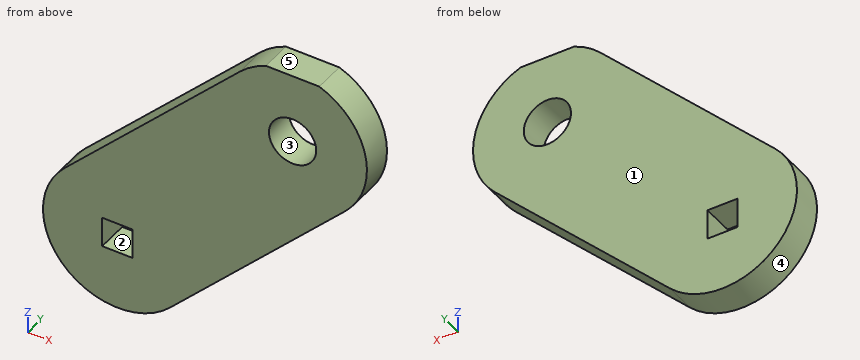
```python
from build123d import *

# Parameters (mm, degrees)
SKETCH2_R           = 4.7625
SKETCH2_W           = 6.1
SKETCH2_H           = 6.1
BOSS_EXTRUDE1_DEPTH = 6.35


with BuildPart() as part:
    # Sketch2 → Boss-Extrude1 (new body)
    with BuildSketch(Plane(origin=(0, 0, 0), x_dir=(1, 0, 0), z_dir=(0, 1, 0))):
        with BuildLine():
            Line((45.961940777, -24.748737342), (10.606601718, 10.606601718))
            ThreePointArc((10.606601718, 10.606601718), (-10.606601718, 10.606601718), (-10.606601718, -10.606601718))
            Line((-10.606601718, -10.606601718), (24.748737342, -45.961940777))
            ThreePointArc((24.748737342, -45.961940777), (27.181420958, -47.93258291), (29.970174252, -49.355339059))
            Line((29.970174252, -49.355339059), (40.740503866, -49.355339059))
            ThreePointArc((40.740503866, -49.355339059), (50.028626393, -38.468960557), (45.961940777, -24.748737342))
        make_face()
        with Locations(Location((35.355339059, -35.355339059, 0), (0, 0, 270))):
            Circle(SKETCH2_R, mode=Mode.SUBTRACT)
        Rectangle(SKETCH2_W, SKETCH2_H, mode=Mode.SUBTRACT)
    extrude(amount=-BOSS_EXTRUDE1_DEPTH)


solid = part.part
```
Could you check a few things on this model? Use its own coordinates, in mm. Face numbers are marked on the shaded views. A direction names the side the tool comes from. Give positions to 0.01 mm unless a question says otherwise; leave off trailing zeros. Loops run counter-clockwise (first coordinate to the right, second up) from the corner with the lowest first, then second, coordinate; pieces in that order, holes last. Notation, with made-up numbers: (83, 89) - (122, 89) arc R21 ccw to (122, 93) - close; hole circle Ø10 at (1.25, 8.5). An arc over 180 degrees is marked (long way). Answer in a Markdown table with one row per item. Add a question column.
Q1. If we section it at D-D (z = 29.5): List the corners of the cut face in (x, y) for me, plus the area to 3 significant figures.
Q2. If we section it at C-C (y = -4.25): State how many separate pieces and enclosed holes the cut face has, plus the area to 3 significant figures.
Q3. Please list where these lines run through material, in increasing order: L1, parallel to Z at x = -0.5, y = -2; L2, parallel to X at y = -3.5, z = 1; L3, parallel to X at y = -5, z = 36. Write a range as from..to.
Q4. If we section it at B-B (z = 0): List the corners of the cut face in (x, y) for me.
Q5. If we section it at A-A (x = 0.5): List the corners of the cut face in (y, z) for me.
Q6. Which directions (+Z, -Z, +X, -X, +Y, -Y) give clear straight access to the entire face, cutting with the end or side of a thin tool? Please do the marked faces 1 and 2.
Q7. For pin 1 (2 mm diameter, centred on y = -3.5, z = -4.5, fed in from -X); pin 2 (1.5 mm diameter, centred on y = -2, z = 5, fed in from +X), each with a flat end and sliding along its axis, tell me the tip position at first contact or that it passes through.
Q8. We'd pull the mould along Z, two halves only. Please class the marked faces 3, 4 and 5: +Z half, -Z half, draft (parallel to the pull), parting line (faces both ways), or undercut.
The answers:
| question | item | result |
|---|---|---|
| 1 | outline | (8.29, -6.35) - (49.17, -6.35) - (49.17, 0) - (8.29, 0) - close |
| 1 | area | 260 mm^2 |
| 2 | separate pieces | 1 |
| 2 | enclosed holes | 2 |
| 2 | area | 2,090 mm^2 |
| 3 | L1 | z = -14.99..-3.05, 3.05..20.71 |
| 3 | L2 | x = -14.97..-3.05, 3.05..22.21 |
| 3 | L3 | x = 14.79..30.64, 40.07..50.34 |
| 4 | outline | (-15, -6.35) - (-3.05, -6.35) - (-3.05, 0) - (-15, 0) - close; (3.05, -6.35) - (21.21, -6.35) - (21.21, 0) - (3.05, 0) - close |
| 5 | outline | (-6.35, -14.99) - (0, -14.99) - (0, -3.05) - (-6.35, -3.05) - close; (-6.35, 3.05) - (0, 3.05) - (0, 21.71) - (-6.35, 21.71) - close |
| 6 | face 1 | +Z, -Z, +X, -X, +Y |
| 6 | face 2 | +Y, -Y |
| 7 | pin 1 | stops at x = -14.59 |
| 7 | pin 2 | stops at x = 26.96 |
| 8 | face 3 | undercut |
| 8 | face 4 | parting line |
| 8 | face 5 | +Z half |
